```python
from build123d import *

# Parameters (mm, degrees)
BOSS_EXTRUDE1_DEPTH      = 350
BOSS_EXTRUDE1_DEPTH_BACK = 350
CUT_EXTRUDE1_DEPTH       = 250
CUT_EXTRUDE1_DEPTH_BACK  = 250


with BuildPart() as part:
    # Sketch6 → Boss-Extrude1 (new, two sides: drawn at the far end of the back side and taken through both)
    with BuildSketch(Plane.XY.offset(-BOSS_EXTRUDE1_DEPTH_BACK)):
        with BuildLine():
            Line((971.509879636, -124.075068782), (-252.203431313, -124.075068782))
            Line((-252.203431313, -124.075068782), (263.900031848, 351.768416645))
            add(Edge.make_bspline(
                [(263.900031848, 351.768416645), (546.111311767, 505.694887208), (815.348837324, 351.768416645)],
                knots=[0, 0, 0, 1, 1, 1], degree=2))
            add(Edge.make_bspline(
                [(815.348837324, 351.768416645), (947.510823837, 130.321252054), (971.509879636, -124.075068782)],
                knots=[0, 0, 0, 1, 1, 1], degree=2))
        make_face()
    extrude(amount=BOSS_EXTRUDE1_DEPTH + BOSS_EXTRUDE1_DEPTH_BACK)

    # Sketch5 → Cut-Extrude1 (cut, two sides: drawn at the far end of the back side and taken through both)
    with BuildSketch(Plane.XY.offset(-CUT_EXTRUDE1_DEPTH_BACK)):
        with BuildLine():
            Line((0, 0), (672.171335821, 0))
            ThreePointArc((672.171335821, 0), (695.015340994, 7.164783727), (709.67572834, 26.092428616))
            Line((709.67572834, 26.092428616), (818.005303321, 318.223584322))
            ThreePointArc((818.005303321, 318.223584322), (820.376071762, 335.288930001), (815.348837324, 351.768416645))
            add(Edge.make_bspline(
                [(263.900031848, 351.768416645), (546.111311767, 505.694887208), (815.348837324, 351.768416645)],
                knots=[0, 0, 0, 1, 1, 1], degree=2))
            Line((263.900031848, 351.768416645), (263.900031848, 166.522987154))
            ThreePointArc((263.900031848, 166.522987154), (258.258035835, 146.04061517), (242.923653745, 131.336316241))
            Line((242.923653745, 131.336316241), (0, 0))
        make_face()
    extrude(amount=CUT_EXTRUDE1_DEPTH + CUT_EXTRUDE1_DEPTH_BACK, mode=Mode.SUBTRACT)


solid = part.part
```
Could you check a few things on this model? Use its own coordinates, in mm. A direction names the side the tool comes from. Give positions to 0.01 mm unless a question says otherwise; leave off trailing zeros. Order: outer loops, then holes, each group sorted by start corner. A loop starts at its lowest first (then second) coordinate and runs counter-clockwise, first axis right, second up.
Q1. For faces 5 (the cylindrical face through (258.41, 146.3, -3.5)), 6 (the cylindrical face through (694.735, 6.972, -3.5)), 7 (the flat face through (2.24, 110.52, -4.9)), which set-ups out of +Z, -Z, +X, -X, +Y, -Y let a thin tool reach every point of the face, with its end or its side?
Q2. Suppose I cut it at B-B, the plane x = -179. Write out the boundary of the cut face in (y, z).
Q3. I'm going to push flat-ended pins straight in: P1, Ø3, axis at x = 483, z = 142, coming from the +Y side; P2, Ø6, axis at y = 208.5, z = -262, coming from the -X side. Where does each tip first touch, or does it pass through?
Q4. Suppose I cut it at A-A, the plane x = 156. Write out the boundary of the cut face in (y, z), and give its area (3 significant figures).
Q5. Suppose I cut it at C-C, the plane x = -39.5. Write out the boundary of the cut face in (y, z), and give its area (3 significant figures).
Q6. If I drill on line 1 along Z through (x, y) = (539, 68); line 2 along Y through (x, z) = (547.5, -242); line 3 along X through (y, z) = (12.5, -124.5), over which ranges is the centre line in solid material (lowest first)?
Q7. We'd pull the mould along Y, two halves only. Please class faces 1 (the flat face through (331, 0, -4)), 2 (the flat face through (368, -124.075, -5)), 3 (the flat face through (263.9, 260, -4)), 4 (the cylindrical face through (820.395, 335.047, -3.5)): +Y half, -Y half, draft (parallel to the pull), parting line (faces both ways), or undercut.
Solution:
1. face 5: none
1. face 6: +Y
1. face 7: +Z, -Z, -X, +Y
2. outline: (-124.08, -350) - (-56.58, -350) - (-56.58, 350) - (-124.08, 350) - close
3. P1: stops at y = 0
3. P2: stops at x = 105.26
4. outline: (-124.08, -350) - (252.29, -350) - (252.29, 350) - (-124.08, 350) - close; hole (0, -250) - (84.34, -250) - (84.34, 250) - (0, 250) - close
4. area: 221,000 mm2
5. outline: (-124.08, -350) - (72.04, -350) - (72.04, 350) - (-124.08, 350) - close
5. area: 137,000 mm2
6. line 1: z = -350 to -250, 250 to 350
6. line 2: y = -124.08 to 0
6. line 3: x = -104.07 to 23.12, 701.22 to 950.32
7. face 1: undercut
7. face 2: -Y half
7. face 3: draft
7. face 4: undercut
